Read the model definition and answer for the solid it produces. Units are mm, in the model's axes. A direction names the side the tool comes from. Give positions to 0.01 mm unless a question says otherwise; leave off trailing zeros. Order: outer loops, then holes, each group sorted by start corner. A loop starts at its lowest first (then second) coordinate and runs counter-clockwise, first axis right, second up. Notation, with made-up numbers: (-17.5, -32) - (27.5, -32) arc R12 cw to (27.5, -24) - close; hole circle Ø1 at (52.5, 46.25). An arc over 180 degrees is marked (long way). Return JSON: item names as keys, results as strings.
```python
from build123d import *

# Parameters (mm, degrees)
EXTRUDE_3_DEPTH     = 2
EXTRUDE_3_2_DEPTH   = 2
SKETCH_2_R          = 3.75
SKETCH_2_R_2        = 2.5
EXTRUDE_5_DEPTH     = 3
SKETCH_3_R          = 3.75
SKETCH_3_R_2        = 2.5
EXTRUDE_6_DEPTH     = 2
SKETCH_4_R          = 0.5
CUT_EXTRUDE_1_DEPTH = 2
SKETCH_5_R          = 2.5
EXTRUDE_7_DEPTH     = 1
SKETCH_6_R          = 2.5
CUT_EXTRUDE_2_DEPTH = 0.5
SKETCH_7_R          = 1.25
CUT_EXTRUDE_3_DEPTH = 5


with BuildPart() as part:
    # Sketch 1 → Extrude 3 (new body)
    with BuildSketch(Plane.XY):
        with BuildLine():
            ThreePointArc((-2.88547071, -2.395111434), (-3.527252129, -1.273182005), (-3.75, 0))
            ThreePointArc((-3.75, 0), (-3.527252129, 1.273182005), (-2.88547071, 2.395111434))
            Line((-2.88547071, 2.395111434), (-14.07082784, 1.998745461))
            ThreePointArc((-14.07082784, 1.998745461), (-16, 0), (-14.07082784, -1.998745461))
            Line((-14.07082784, -1.998745461), (-2.88547071, -2.395111434))
        make_face()
    extrude(amount=EXTRUDE_3_DEPTH)



with BuildPart() as body_2:
    # Sketch 1 → Extrude 3 2 (new body)
    with BuildSketch(Plane.XY):
        with BuildLine():
            Line((14.07082784, 1.998745461), (2.88547071, 2.395111434))
            ThreePointArc((2.88547071, 2.395111434), (3.75, 0), (2.88547071, -2.395111434))
            Line((2.88547071, -2.395111434), (14.07082784, -1.998745461))
            ThreePointArc((14.07082784, -1.998745461), (16, 0), (14.07082784, 1.998745461))
        make_face()
    extrude(amount=EXTRUDE_3_2_DEPTH)


with BuildPart() as body_3:
    # Sketch 2 → Extrude 5 (new body)
    with BuildSketch(Plane.XY.offset(2)):
        Circle(SKETCH_2_R)
        Circle(SKETCH_2_R_2, mode=Mode.SUBTRACT)
    extrude(amount=EXTRUDE_5_DEPTH)


with BuildPart() as part_1:
    add(part.part)

    add(body_2.part)  # Extrude 6 merges body 2

    add(body_3.part)  # Extrude 6 merges body 3
    # Sketch 3 → Extrude 6 (add)
    with BuildSketch(Plane(origin=(0, 0, 2), x_dir=(-1, 0, 0), z_dir=(0, 0, -1))):
        Circle(SKETCH_3_R)
        Circle(SKETCH_3_R_2, mode=Mode.SUBTRACT)
    extrude(amount=EXTRUDE_6_DEPTH)

    # Sketch 4 → Cut-Extrude 1 (cut)
    with BuildSketch(Plane(origin=(0, 0, 0), x_dir=(-1, 0, 0), z_dir=(0, 0, -1))):
        with Locations((-14.5, 0)):
            Circle(SKETCH_4_R)
        with Locations((-4.5, 0)):
            Circle(SKETCH_4_R)
        with Locations((-6.5, 0)):
            Circle(SKETCH_4_R)
        with Locations((-8.5, 0)):
            Circle(SKETCH_4_R)
        with Locations((-10.5, 0)):
            Circle(SKETCH_4_R)
        with Locations((-12.5, 0)):
            Circle(SKETCH_4_R)
        with Locations((4.5, 0)):
            Circle(SKETCH_4_R)
        with Locations((6.5, 0)):
            Circle(SKETCH_4_R)
        with Locations((8.5, 0)):
            Circle(SKETCH_4_R)
        with Locations((10.5, 0)):
            Circle(SKETCH_4_R)
        with Locations((12.5, 0)):
            Circle(SKETCH_4_R)
        with Locations((14.5, 0)):
            Circle(SKETCH_4_R)
    extrude(amount=-CUT_EXTRUDE_1_DEPTH, mode=Mode.SUBTRACT)

    # Sketch 5 → Extrude 7 (add)
    with BuildSketch(Plane(origin=(0, 0, 0), x_dir=(-1, 0, 0), z_dir=(0, 0, -1))):
        Circle(SKETCH_5_R)
    extrude(amount=-EXTRUDE_7_DEPTH)

    # Sketch 6 → Cut-Extrude 2 (cut)
    with BuildSketch(Plane(origin=(0, 0, 0), x_dir=(-1, 0, 0), z_dir=(0, 0, -1))):
        Circle(SKETCH_6_R)
    extrude(amount=-CUT_EXTRUDE_2_DEPTH, mode=Mode.SUBTRACT)

    # Sketch 7 → Cut-Extrude 3 (cut)
    with BuildSketch(Plane(origin=(0, 0, 0.5), x_dir=(-1, 0, 0), z_dir=(0, 0, -1))):
        Circle(SKETCH_7_R)
    extrude(amount=-CUT_EXTRUDE_3_DEPTH, mode=Mode.SUBTRACT)


solid = part_1.part
```
Q1. For faces 4 (the flat face through (1, -1, 0.5)), 5 (the cylindrical face through (0.27, -1.22, 0.75)), 6 (the flat face through (1, -1, 1)), determine the directions among +Z, -Z, +X, -X, +Y, -Y from which every point of the face is accessible in a straight line to the end or side of a thin tool.
Values:
{"face 4": "-Z", "face 5": "+Z, -Z", "face 6": "+Z"}
Q2. A cutting plane is placed at C-C (x = 8.5). Write down the section's boundary in (y, z), and give its area (3 significant figures).
Values:
{"outline": "(-2.2, 0) - (-0.5, 0) - (-0.5, 2) - (-2.2, 2) - close; (0.5, 0) - (2.2, 0) - (2.2, 2) - (0.5, 2) - close", "area": "6.78 mm²"}
Q3. A cutting plane is placed at B-B (z = 4.05). Write down the section's boundary in (x, y).
Values:
{"outline": "circle Ø7.5 at (0, 0); hole circle Ø5 at (0, 0)"}
Q4. Determine the mould class of faces 1 (the cylindrical face through (0.54, -2.44, 0.25)), 2 (the cylindrical face through (-4, 0, 1)), 3 (the flat face through (0, 3, 5)) for opening direction X: released by +X, released by -X, zero draft, split by the parting line, or undercut.
Values:
{"face 1": "undercut", "face 2": "undercut", "face 3": "zero draft"}
Q5. Consider L1, parallel to Y at x = 0, z = 1.35; L2, parallel to Y at x = -10.5, z = 0.5; L3, parallel to X at y = 1, z = 2.35. Determine where each line is inside the solid, lowest interval first.
Values:
{"L1": "y = -3.75 to -2.5, 2.5 to 3.75", "L2": "y = -2.13 to -0.5, 0.5 to 2.13", "L3": "x = -3.61 to -2.29, 2.29 to 3.61"}
Q6. A cutting plane is placed at A-A (x = 14.5). Write down the section's boundary in (y, z).
Values:
{"outline": "(-1.94, 0) - (-0.5, 0) - (-0.5, 2) - (-1.94, 2) - close; (0.5, 0) - (1.94, 0) - (1.94, 2) - (0.5, 2) - close"}
Q7. Given pin 1 (1.5 mm diameter, centred on x = -6, z = 0.5, fed in from +Y); pin 2 (2 mm diameter, centred on x = -8, y = -1.5, fed in from +Z), each flat-ended and moving along its own axis, determine where each tip first touches the part or whether it passes through.
Values:
{"pin 1": "stops at y = 2.31", "pin 2": "stops at z = 2"}
